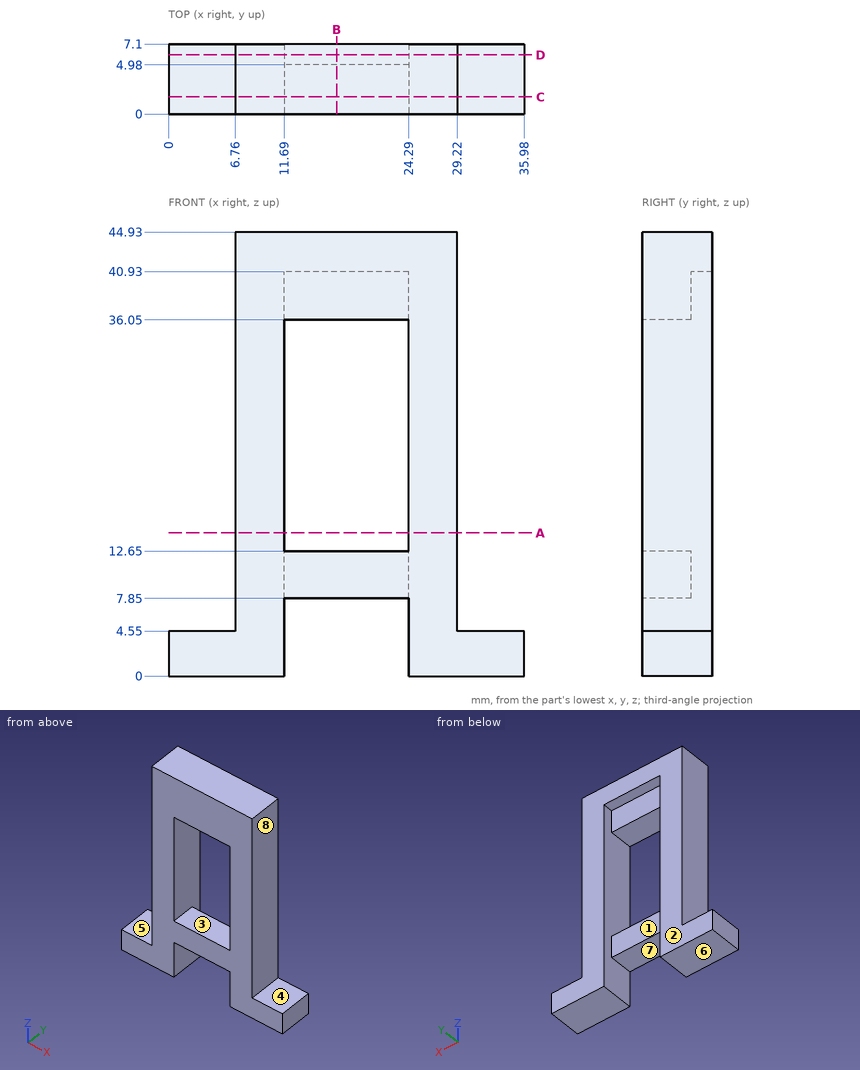
Geometry check sheet. Reference: drawing and pictorial views, mm from the part's lowest x, y, z. A direction names the side the tool comes from. Coordinates: 2 decimals unless noted, no trailing zeros. Write each loop counter-clockwise with the first axis right and the second up, starting at its lowest first coordinate (ties: lowest second). Pieces come first, ordered by that corner, then holes. Notation, with made-up numbers: M -17.75,81.25 L 27.25,81.25 A21 cw 27.25,89.25 Z; hole C 36.5,-1 d7. An arc over 180 degrees is marked long. Write item = value, one per line. Start each with the question number.
1. Sectioned sample at A-A (z = 14.5). Record the cut outline in (x, y), then the cut area to 3 significant figures.
2. Sectioned sample at C-C (y = 1.75). Record the cut outline in (x, z).
3. Thickness scan on probe 1 along Z at (x, y) = (19.5, 4.25); probe 2 along X at (y, z) = (4.5, 19); probe 3 along Z at (x, y) = (3, 0.5). Record the ranges inside material, lowest first.
4. Go/stop test with flat-tipped pins: pin 1 (2 mm diameter, centred on x = 2, y = 4.5, fed in from +Z); pin 2 (2.5 mm diameter, centred on x = 17.5, y = 3, fed in from -Z); pin 3 (2.5 mm diameter, centred on x = 19, z = 39, fed in from +Y). Record where each tip stops, or that it passes through.
5. Mould release check, pull along X, two halves, no side actions. Record for the marked faces 6, 7 and 8: pulls with the +X half, pulls with the -X half, needs draft (parallel to the pull), parting line crosses it, or undercut.
6. Sectioned sample at B-B (x = 17). Record the cut outline in (y, z).
7. Sectioned sample at D-D (y = 6). Record the cut outline in (x, z).
8. Tool access check on the marked faces 1, 2, 3, 4 and 5. Record the directions out of +Z, -Z, +X, -X, +Y, -Y that give a thin tool (end or side, any length) a straight path to the whole face; none if there is none.
The answers:
q1.outline = M 6.76,0 L 11.69,0 L 11.69,7.1 L 6.76,7.1 Z; M 24.29,0 L 29.22,0 L 29.22,7.1 L 24.29,7.1 Z
q1.area = 70.0 mm²
q2.outline = M 0,0 L 11.69,0 L 11.69,7.85 L 24.29,7.85 L 24.29,0 L 35.98,0 L 35.98,4.55 L 29.22,4.55 L 29.22,44.93 L 6.76,44.93 L 6.76,4.55 L 0,4.55 Z; hole M 11.69,12.65 L 24.29,12.65 L 24.29,36.05 L 11.69,36.05 Z
q3.probe_1 = 7.85 to 12.65, 36.05 to 44.93
q3.probe_2 = 6.76 to 11.69, 24.29 to 29.22
q3.probe_3 = 0 to 4.55
q4.pin_1 = 4.55
q4.pin_2 = 7.85
q4.pin_3 = 4.98
q5.face_6 = needs draft
q5.face_7 = undercut
q5.face_8 = pulls with the +X half
q6.outline = M 0,7.85 L 4.98,7.85 L 4.98,12.65 L 0,12.65 Z; M 0,36.05 L 4.98,36.05 L 4.98,40.93 L 7.1,40.93 L 7.1,44.93 L 0,44.93 Z
q7.outline = M 0,0 L 11.69,0 L 11.69,40.93 L 24.29,40.93 L 24.29,0 L 35.98,0 L 35.98,4.55 L 29.22,4.55 L 29.22,44.93 L 6.76,44.93 L 6.76,4.55 L 0,4.55 Z
q8.face_1 = -Z, +Y
q8.face_2 = +Z, -Z, +X, -X, +Y
q8.face_3 = +Y, -Y
q8.face_4 = +Z, +X, +Y, -Y
q8.face_5 = +Z, -X, +Y, -Y
